Design review of the part built by this model. Coordinates are the model's own, in mm. Face numbers are marked on the shaded views. Round coordinates to 2 decimals unless told otherwise and drop trailing zeros. Write each loop counter-clockwise with the first axis right and the second up, starting at its lowest first coordinate (ties: lowest second). Pieces come first, ordered by that corner, then holes. Notation, with made-up numbers: (-23, -13) -> (11, -13) arc R24 ccw to (11, 18) -> close; hole circle Ø7 at (35.5, 65.25). An arc over 180 degrees is marked (long way). One line per question, with ' | ' between items. Start each with the question number.
1) Mouldability with a two-part tool opening along X and no side actions: class the marked faces 1, 2 and 3 as +X half, -X half, draft (parallel to the pull), parting line (faces both ways), or undercut.
2) Consider section A-A (y = 45.5). Give the boundary of the cut face in (x, z), then the cut area to 3 significant figures.
3) Consider section C-C (x = -15). Give the boundary of the cut face in (y, z).
4) Insertion check: pin 1 Ø3 at (x, z) = (60, -117.5) entering from -Y; pin 2 Ø12 at (x, y) = (4, 44) entering from +Z; pin 3 Ø10 at (y, z) = (53, -76) entering from -X. Each pin has a flat end and moves straight along its axis. Give the tip position at first contact, or say it passes through.
5) Consider section B-B (z = -79). Give the boundary of the cut face in (x, y), then the cut area to 3 significant figures.
6) For probe 1 along X at (y, z) = (39.25, -19); probe 2 along Y at (x, z) = (-66, -69); probe 3 along X at (y, z) = (33.25, -9), list the stretches that pass through material, from the lowest coordinate up.
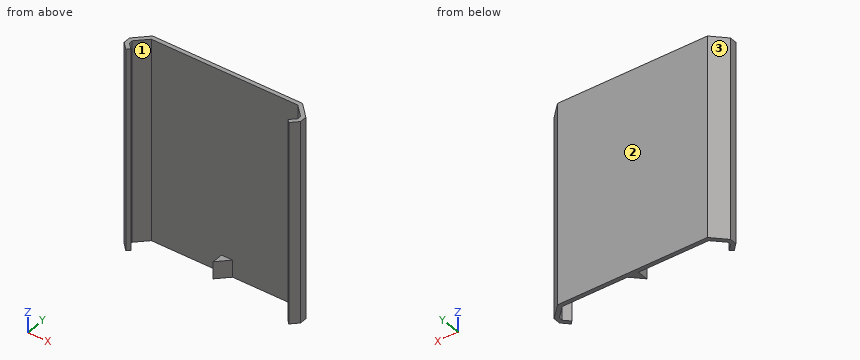
```python
from build123d import *

# Parameters (mm, degrees)
EXTRUDE_1_DEPTH   = 200
EXTRUDE_1_2_DEPTH = 17


with BuildPart() as part:
    # 草图1 → Extrude 1 (new body)
    with BuildSketch(Plane.XY):
        Polygon((78, 32), (83.5, 37.5), (83.5, 41.207106781), (72.707106781, 52), (-72.707106781, 52), (-83.5, 41.207106781), (-83.5, 37.5), (-78, 32), (-80.828427125, 29.171572875), (-87.5, 35.843145751), (-87.5, 42.863961031), (-74.363961031, 56), (74.363961031, 56), (87.5, 42.863961031), (87.5, 35.843145751), (80.828427125, 29.171572875), align=None)
    extrude(amount=-EXTRUDE_1_DEPTH)

    # 草图2 → Extrude 1 2 (add)
    with BuildSketch(Plane(origin=(0, 0, -200), x_dir=(-1, 0, 0), z_dir=(0, 0, -1))):
        Polygon((-7.989949494, 52), (3, 52), (3, 41.010050506), align=None)
    extrude(amount=-EXTRUDE_1_2_DEPTH)


solid = part.part
```
From the geometry:
1) face 1: undercut | face 2: draft | face 3: -X half
2) outline: (-84.86, -200) -> (-79.21, -200) -> (-79.21, 0) -> (-84.86, 0) -> close; (-3, -200) -> (1.49, -200) -> (1.49, -183) -> (-3, -183) -> close; (79.21, -200) -> (84.86, -200) -> (84.86, 0) -> (79.21, 0) -> close | area: 2,340 mm2
3) outline: (52, -200) -> (56, -200) -> (56, 0) -> (52, 0) -> close
4) pin 1: stops at y = 52 | pin 2: stops at z = -183 | pin 3: stops at x = -82.36
5) outline: (-87.5, 35.84) -> (-80.83, 29.17) -> (-78, 32) -> (-83.5, 37.5) -> (-83.5, 41.21) -> (-72.71, 52) -> (72.71, 52) -> (83.5, 41.21) -> (83.5, 37.5) -> (78, 32) -> (80.83, 29.17) -> (87.5, 35.84) -> (87.5, 42.86) -> (74.36, 56) -> (-74.36, 56) -> (-87.5, 42.86) -> close | area: 835 mm2
6) probe 1: x = -87.5 to -83.5, 83.5 to 87.5 | probe 2: y = 52 to 56 | probe 3: x = -84.91 to -79.25, 79.25 to 84.91
